from build123d import *

# Parameters (mm, degrees)
EXTRUDE_1_DEPTH     = 200
SKETCH_2_W          = 200
SKETCH_2_H          = 97.057417657
EXTRUDE_2_DEPTH     = 46.061398085
SKETCH_3_W          = 200
SKETCH_3_H          = 97.057417639
EXTRUDE_3_DEPTH     = 46.061398049
HOLE_WIZARD_1_D     = 50
HOLE_WIZARD_2_D     = 14
HOLE_WIZARD_2_DEPTH = 30
HOLE_WIZARD_2_TIP   = 4.206024333
CHAMFER_1_SIZE      = 3


with BuildPart() as part:
    # 草图1 → 凸台-拉伸1 (new body)
    with BuildSketch(Plane.XY.offset(100)):
        with BuildLine():
            Line((80.000000036, 0), (80.000000036, 150))
            Line((80.000000036, 150), (-80.000000036, 150))
            Line((-80.000000036, 150), (-80.000000036, 0))
            ThreePointArc((-80.000000036, 0), (0, -80.000000036), (80.000000036, 0))
        make_face()
    extrude(amount=-EXTRUDE_1_DEPTH)

    # 草图2 → 凸台-拉伸2 (add)
    with BuildSketch(Plane(origin=(80.000000036, 0, 0), x_dir=(0, 0, -1), z_dir=(1, 0, 0))):
        with Locations((0, 101.471291153)):
            Rectangle(SKETCH_2_W, SKETCH_2_H)
    extrude(amount=EXTRUDE_2_DEPTH)

    # 草图3 → 凸台-拉伸3 (add)
    with BuildSketch(Plane.ZY.offset(80.000000036)):
        with Locations((0, 101.471291181)):
            Rectangle(SKETCH_3_W, SKETCH_3_H)
    extrude(amount=EXTRUDE_3_DEPTH)

    # 孔1 (through all)
    with Locations(Plane.XY.offset(100)):
        with Locations((0, 0)):
            Hole(HOLE_WIZARD_1_D / 2)

    # 孔2
    with Locations(Plane(origin=(0, 150, 0), x_dir=(1, 0, 0), z_dir=(0, 1, 0))):
        with Locations((-70.811035645, 51.091167344), (-70.811035645, -57.320629237), (90.685157882, -57.320629237), (90.685157882, 51.091167344)):
            Hole(HOLE_WIZARD_2_D / 2, depth=HOLE_WIZARD_2_DEPTH)
            with Locations((0, 0, -(HOLE_WIZARD_2_DEPTH + HOLE_WIZARD_2_TIP / 2))):  # 118° drill point
                Cone(0, HOLE_WIZARD_2_D / 2, HOLE_WIZARD_2_TIP, mode=Mode.SUBTRACT)

    # 倒角1
    chamfer_1_edges = [part.edges().sort_by_distance(p)[0] for p in [
        (97.685157882, 150, -51.091167344),
        (97.685157882, 150, 57.320629237),
        (-63.811035645, 150, 57.320629237),
        (-63.811035645, 150, -51.091167344),
    ]]
    chamfer(chamfer_1_edges, length=CHAMFER_1_SIZE)


solid = part.part
Check sheet for the modelled part. Datum: model origin and axes. Units: mm. A direction names the side the tool comes from. Round coordinates to 2 decimals unless told otherwise and drop trailing zeros. Loops run counter-clockwise (first coordinate to the right, second up) from the corner with the lowest first, then second, coordinate; pieces in that order, holes last. Notation, with made-up numbers: M -11.5,-4 L 15.5,-4 A20 cw 15.5,19 Z; hole C -31,-33.75 d2. An arc over 180 degrees is marked long. One line per item, written item: value.
(1) Thickness scan on line 1 (Y direction, x = 0, z = -39.5); line 2 (Y direction, x = 112, z = -59); line 3 (Y direction, x = -52, z = 85). Record the ranges inside material, lowest first.
Computed values:
line 1: y = -80 to -25, 25 to 150
line 2: y = 52.94 to 150
line 3: y = -60.79 to 150
(2) Release check for a two-part mould opening along X. For faces 4 (the face through (126.061, 102, 1)), 5 (the face through (-77.412, 147.146, -48.354)), 6 (the face through (-80, 27, 1)) record: +X half, -X half, draft (parallel to the pull), parting line (faces both ways), or undercut.
Computed values:
face 4: +X half
face 5: undercut
face 6: -X half
(3) Sectioned sample at B-B, the plane y = -12. Record the cut outline in (x, z).
Computed values:
outline: M -79.09,-100 L -21.93,-100 L -21.93,100 L -79.09,100 Z; M 21.93,-100 L 79.09,-100 L 79.09,100 L 21.93,100 Z
(4) Sectioned sample at C-C, the plane z = 37.5. Record the cut outline in (x, y), then the cut area to 3 significant figures.
Computed values:
outline: M -126.06,52.94 L -80,52.94 L -80,0 A80 ccw 80,0 L 80,52.94 L 126.06,52.94 L 126.06,150 L -126.06,150 Z; hole C 0,0 d50
area: 41,000 mm^2
(5) Sectioned sample at D-D, the plane y = 43. Record the cut outline in (x, z).
Computed values:
outline: M -80,-100 L 80,-100 L 80,100 L -80,100 Z
(6) Depth check by flat-ended pin: pin 1 Ø16 at (x, z) = (-70.81, -51.09) entering from +Y; pin 2 Ø4 at (y, z) = (1, 4.5) entering from +X; pin 3 Ø18 at (x, z) = (90.69, -51.09) entering from -Y; pin 4 Ø22.5 at (x, z) = (90.69, 57.32) entering from +Y. Enter the tip coordinate at first touch or a pass-through.
Computed values:
pin 1: stops at y = 148
pin 2: stops at x = 80
pin 3: stops at y = 52.94
pin 4: stops at y = 150
(7) Sectioned sample at A-A, the plane x = 0. Record the cut outline in (y, z), then the cut area to 3 significant figures.
Computed values:
outline: M -80,-100 L -25,-100 L -25,100 L -80,100 Z; M 25,-100 L 150,-100 L 150,100 L 25,100 Z
area: 36,000 mm^2
(8) Access from +Z, -Z, +X, -X, +Y, -Y to the whole of each face (thin tool, end or side, straight path). Record for faces 1 (the face through (80, 26, 1)), 2 (the face through (96.24, 133.31, -46.83)), 3 (the face through (-103, 52.943, -1)).
Computed values:
face 1: +Z, -Z, +X, -Y
face 2: +Y
face 3: +Z, -Z, -X, -Y
